```python
from build123d import *

# Parameters (mm, degrees)
BOSS_EXTRUDE1_DEPTH = 5
SKETCH2_R           = 9
CUT_EXTRUDE1_DEPTH  = 4
SKETCH3_R           = 7.75
CUT_EXTRUDE2_DEPTH  = 15
SKETCH4_R           = 4
CUT_EXTRUDE3_DEPTH  = 15
SKETCH5_R           = 1.55
CUT_EXTRUDE4_DEPTH  = 15
SKETCH6_R           = 2.6
CUT_EXTRUDE5_DEPTH  = 15
CUT_EXTRUDE7_DEPTH  = 15
CUT_EXTRUDE8_DEPTH  = 10
SKETCH9_R           = 2.75
CUT_EXTRUDE10_DEPTH = 2.8
BOSS_EXTRUDE2_DEPTH = 5


with BuildPart() as part:
    # Sketch1 → Boss-Extrude1 (new body)
    with BuildSketch(Plane.XY):
        with BuildLine():
            Line((0, 11.5), (120, 11.5))
            ThreePointArc((120, 11.5), (131.5, 0), (120, -11.5))
            Line((120, -11.5), (0, -11.5))
            ThreePointArc((0, -11.5), (-11.5, 0), (0, 11.5))
        make_face()
    extrude(amount=-BOSS_EXTRUDE1_DEPTH)

    # Sketch2 → Cut-Extrude1 (cut)
    with BuildSketch(Plane.XY):
        with Locations((120, 0)):
            Circle(SKETCH2_R)
    extrude(amount=-CUT_EXTRUDE1_DEPTH, mode=Mode.SUBTRACT)

    # Sketch3 → Cut-Extrude2 (cut)
    with BuildSketch(Plane.XY):
        with Locations((120, 0)):
            Circle(SKETCH3_R)
    extrude(amount=-CUT_EXTRUDE2_DEPTH, mode=Mode.SUBTRACT)

    # Sketch4 → Cut-Extrude3 (cut)
    with BuildSketch(Plane.XY):
        Circle(SKETCH4_R)
    extrude(amount=-CUT_EXTRUDE3_DEPTH, mode=Mode.SUBTRACT)

    # Sketch5 → Cut-Extrude4 (cut)
    with BuildSketch(Plane.XY):
        with Locations((0, 8)):
            Circle(SKETCH5_R)
        with Locations((0, -8)):
            Circle(SKETCH5_R)
    extrude(amount=-CUT_EXTRUDE4_DEPTH, mode=Mode.SUBTRACT)

    # Sketch6 → Cut-Extrude5 (cut)
    with BuildSketch(Plane.XY):
        with Locations((-9.5, 0)):
            Circle(SKETCH6_R)
        with Locations((9.5, 0)):
            Circle(SKETCH6_R)
    extrude(amount=-CUT_EXTRUDE5_DEPTH, mode=Mode.SUBTRACT)

    # Sketch8 → Cut-Extrude7 (cut)
    with BuildSketch(Plane.XY):
        with BuildLine():
            ThreePointArc((103.5, -8.220260856), (106.328427125, -7.048687981), (107.5, -4.220260856))
            Line((107.5, -4.220260856), (107.5, 3.779739144))
            ThreePointArc((107.5, 3.779739144), (106.328427125, 6.608166269), (103.5, 7.779739144))
            Line((103.5, 7.779739144), (61.5, 7.779739144))
            Line((61.5, 7.779739144), (77.5, -8.220260856))
            Line((77.5, -8.220260856), (103.5, -8.220260856))
        make_face()
        with BuildLine():
            Line((35.5, -8.220260856), (19.5, 7.779739144))
            ThreePointArc((19.5, 7.779739144), (16.722169997, 6.581192541), (15.578063312, 3.780500952))
            Line((15.578063312, 3.780500952), (15.578063312, -4.220260856))
            ThreePointArc((15.578063312, -4.220260856), (16.749636187, -7.048687981), (19.578063312, -8.220260856))
            Line((19.578063312, -8.220260856), (35.5, -8.220260856))
        make_face()
    extrude(amount=-CUT_EXTRUDE7_DEPTH, mode=Mode.SUBTRACT)

    # Sketch8<3> → Cut-Extrude8 (cut)
    with BuildSketch(Plane.XY):
        Polygon((40.5, -8.220260856), (56.5, 7.779739144), (24.5, 7.779739144), align=None)
        Polygon((77.5, -8.220260856), (61.5, 7.779739144), (45.5, -8.220260856), align=None)
    extrude(amount=-CUT_EXTRUDE8_DEPTH, mode=Mode.SUBTRACT)

    # Sketch9 → Cut-Extrude10 (cut)
    with BuildSketch(Plane(origin=(0, 0, -5), x_dir=(-1, 0, 0), z_dir=(0, 0, -1))):
        with Locations((0, 8)):
            Circle(SKETCH9_R)
        with Locations((0, -8)):
            Circle(SKETCH9_R)
    extrude(amount=-CUT_EXTRUDE10_DEPTH, mode=Mode.SUBTRACT)

    # Sketch8<4> → Boss-Extrude2 (add)
    with BuildSketch(Plane.XY):
        Polygon((82.5, -8.220260856), (66.5, 7.779739144), (61.5, 7.779739144), (77.5, -8.220260856), align=None)
        Polygon((87.5, -8.220260856), (103.5, 7.779739144), (98.5, 7.779739144), (82.5, -8.220260856), align=None)
    extrude(amount=-BOSS_EXTRUDE2_DEPTH)


solid = part.part
```
Build history of the part. All positions in model axes, mm. A direction names the side the tool comes from. Coordinates: 2 decimals unless noted, no trailing zeros. Write each loop counter-clockwise with the first axis right and the second up, starting at its lowest first coordinate (ties: lowest second). Pieces come first, ordered by that corner, then holes.
1. Drill centre lines: probe 1 along Y at (x, z) = (0, -3.8); probe 2 along Y at (x, z) = (0, -1.15); probe 3 along Y at (x, z) = (120, -2.6). Where is each one in solid material? Low to high.
Answer block:
probe 1: y = -11.5 to -10.75, -5.25 to -4, 4 to 5.25, 10.75 to 11.5
probe 2: y = -11.5 to -9.55, -6.45 to -4, 4 to 6.45, 9.55 to 11.5
probe 3: y = -11.5 to -9, 9 to 11.5
2. Band-saw the part on B-B, the plane x = 9.5. Give the cut face in (y, z).
Answer block:
outline: (-11.5, -5) - (-2.6, -5) - (-2.6, 0) - (-11.5, 0) - close; (2.6, -5) - (11.5, -5) - (11.5, 0) - (2.6, 0) - close
3. Drop a flat-ended pin along its axis: pin 1 (1.6 mm diameter, centred on x = 1, y = -8, fed in from -Z). Give the stop position or say it passes through.
Answer block:
pin 1: stops at z = -2.2
4. Band-saw the part on C-C, the plane x = -9.5. Give the cut face in (y, z).
Answer block:
outline: (-6.48, -5) - (-2.6, -5) - (-2.6, 0) - (-6.48, 0) - close; (2.6, -5) - (6.48, -5) - (6.48, 0) - (2.6, 0) - close
5. 3-axis set-ups, long thin cutter, end or side, ignore diameter. For faces 4 (the flat face through (43, 8, 0)), 5 (the cylindrical face through (0.596, 5.315, -3.62)), 6 (the cylindrical face through (16.75, 6.61, -2.46)), 7 (the flat face through (124, 7, -4)): which of +Z, -Z, +X, -X, +Y, -Y reach the whole face in a straight line?
Answer block:
face 4: +Z, +X, -X, +Y, -Y
face 5: -Z
face 6: +Z, -Z
face 7: +Z
6. Band-saw the part on A-A, the plane z = -2.95. Give the number of separate pieces and of enclosed holes in the cut face, and give its area (3 significant figures).
Answer block:
separate pieces: 1
enclosed holes: 10
area: 1,650 mm2
7. Pull direction Y, two halves, no side cores. Call faces 1 (the cylindrical face through (106.297, -7.08, -2.465)), 2 (the flat face through (43, 8, -5)), 3 (the flat face through (61, -11.5, -2)): released by +Y, released by -Y, zero draft, split by the parting line, or undercut.
Answer block:
face 1: undercut
face 2: zero draft
face 3: released by -Y
